Verification items for the finished model (mm, model axes). A direction names the side the tool comes from. Round coordinates to 2 decimals unless told otherwise and drop trailing zeros. Loops run counter-clockwise (first coordinate to the right, second up) from the corner with the lowest first, then second, coordinate; pieces in that order, holes last. Notation, with made-up numbers: (46, 25) -> (57, 25) arc R9 ccw to (57, 39) -> close; hole circle Ø7 at (21, 16). An arc over 180 degrees is marked (long way). Write item = value, one per line. Start each with the question number.
```python
from build123d import *

# Parameters (mm, degrees)
F0_R     = 2.5
F1_DEPTH = 7
F2_R     = 3.6213085246
F3_DEPTH = 7.5
F5_DEPTH = 12.5
F6_SIZE  = 1
F7_R     = 1.7235477432
F8_DEPTH = 4.57
F8_TAPER = 5


with BuildPart() as f1:
    # F0 (on Top) → F1 (new body)
    with BuildSketch(Plane.XY):
        Circle(F0_R)
    extrude(amount=F1_DEPTH)

    # F2 (on Front) → F3 (join, symmetric)
    with BuildSketch(Plane.XZ):
        with Locations((0, 6.4717903733)):
            Circle(F2_R)
    extrude(amount=F3_DEPTH, both=True)

    # F4 (on Right) → F5 (cut, symmetric)
    with BuildSketch(Plane.YZ):
        with BuildLine():
            ThreePointArc((0, 10.2597363293), (4.7557858598, 8.1323980884), (7.9216584563, 3.9947275072))
            Line((7.9216584563, 3.9947275072), (7.9610617831, 10.2597363293))
            Line((7.9610617831, 10.2597363293), (0, 10.2597363293))
        make_face()
    extrude(amount=F5_DEPTH, both=True, mode=Mode.SUBTRACT)

    # F6
    f6_edges = [f1.edges().sort_by_distance(p)[0] for p in [
        (-3.621309, -7.5, 6.47179),
    ]]
    chamfer(f6_edges, length=F6_SIZE)

    # F7 (on face) → F8 (join)
    with BuildSketch(Plane.XZ.offset(7.5)):
        with Locations((0, 6.4717903733)):
            Circle(F7_R)
    extrude(amount=F8_DEPTH, taper=F8_TAPER)


solid = f1.part
```
(1) Section check D-D on y = -3.75. Enter the section's corners in (x, z).
(2) Access from +Z, -Z, +X, -X, +Y, -Y to the whole of each face (thin tool, end or side, straight path). Record for faces 1 (the flat face through (0, -12.07, 6)), 2 (the flat face through (2, -7.5, 6)), 3 (the cylindrical face through (2.385, 0.751, 1.471)).
(3) Scan lines: line 1 (Z direction, x = 2.5, y = -4.25); line 2 (Y direction, x = 1, z = 4.5); line 3 (X direction, y = 2, z = 1.25). Record each from-to range of solid material in increasing order. Write a range as [from, to].
(4) Section check B-B on y = 0. Enter the section's corners in (x, z).
(5) Section check C-C on z = 1. Enter the section's corners in (x, y).
(6) Depth check by flat-ended pin: pin 1 Ø1 at (y, z) = (2, 2) entering from +X; pin 2 Ø6 at (y, z) = (2, 2) entering from +X; pin 3 Ø1 at (x, y) = (3, -5) entering from +Z. Enter the tip coordinate at first touch or a pass-through.
(7) Section check A-A on x = 0. Enter the section's corners in (y, z), then the cut area to 3 significant figures.
Computed values:
q1.outline = circle Ø7.24 at (0, 6.47)
q2.face_1 = +Z, -Z, +X, -X, -Y
q2.face_2 = -Y
q2.face_3 = -Z
q3.line_1 = [3.85, 9.09]
q3.line_2 = [-7.5, 7.5]
q3.line_3 = [-1.5, 1.5]
q4.outline = (-2.5, 0) -> (2.5, 0) -> (2.5, 3.85) arc R3.62 ccw (long way) to (-2.5, 3.85) -> close
q5.outline = circle Ø5 at (0, 0)
q6.pin_1 = 2
q6.pin_2 = 3.31
q6.pin_3 = 9.09
q7.outline = (-12.07, 5.15) -> (-7.5, 4.75) -> (-7.5, 3.85) -> (-6.5, 2.85) -> (-2.5, 2.85) -> (-2.5, 0) -> (2.5, 0) -> (2.5, 2.85) -> (7.5, 2.85) -> (7.5, 4.87) arc R10.59 ccw to (0.78, 10.09) -> (-6.5, 10.09) -> (-7.5, 9.09) -> (-7.5, 8.2) -> (-12.07, 7.8) -> close
q7.area = 123 mm²
